```python
from build123d import *

# Parameters (mm, degrees)
SKETCH2_W                = 45
SKETCH2_H                = 62
BOSS_EXTRUDE1_DEPTH      = 5
BOSS_EXTRUDE2_DEPTH      = 10
BOSS_EXTRUDE2_DEPTH_BACK = 5
SKETCH3_W                = 55
SKETCH3_H                = 72
SKETCH3_W_2              = 45
SKETCH3_H_2              = 62
FILLET1_R                = 10


with BuildPart() as part:
    # Sketch2 → Boss-Extrude1 (new body)
    with BuildSketch(Plane(origin=(0, 0, 0), x_dir=(1, 0, 0), z_dir=(0, 1, 0))):
        with Locations((22.5, 31)):
            Rectangle(SKETCH2_W, SKETCH2_H)
    extrude(amount=BOSS_EXTRUDE1_DEPTH)

    # Sketch3 → Boss-Extrude2 (add, two sides: drawn at the far end of the back side and taken through both)
    with BuildSketch(Plane(origin=(0, 5, 0), x_dir=(1, 0, 0), z_dir=(0, 1, 0)).offset(-BOSS_EXTRUDE2_DEPTH_BACK)):
        with Locations((22.5, 31)):
            Rectangle(SKETCH3_W, SKETCH3_H)
        with Locations((22.5, 31)):
            Rectangle(SKETCH3_W_2, SKETCH3_H_2, mode=Mode.SUBTRACT)
    extrude(amount=BOSS_EXTRUDE2_DEPTH + BOSS_EXTRUDE2_DEPTH_BACK)

    # Fillet1
    fillet1_edges = [part.edges().sort_by_distance(p)[0] for p in [
        (50, 7.5, 5),
        (-5, 7.5, 5),
        (-5, 7.5, -67),
        (50, 7.5, -67),
    ]]
    fillet(fillet1_edges, radius=FILLET1_R)


solid = part.part
```
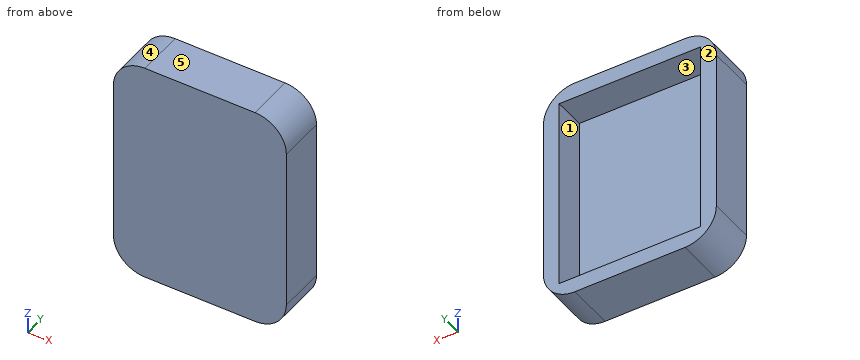
For this review, take the finished solid that the model builds, in its own axes (mm). Face numbers are marked on the shaded views. A direction names the side the tool comes from. Round coordinates to 2 decimals unless told otherwise and drop trailing zeros. Loops run counter-clockwise (first coordinate to the right, second up) from the corner with the lowest first, then second, coordinate; pieces in that order, holes last.
(1) We need section D-D (z = -63). Give the boundary of the cut face in (x, y).
Returned:
outline: (-3, 0) - (48, 0) - (48, 15) - (-3, 15) - close
(2) We need section A-A (y = 10.75). Give the boundary of the cut face in (x, z).
Returned:
outline: (-5, -57) arc R10 ccw to (5, -67) - (40, -67) arc R10 ccw to (50, -57) - (50, -5) arc R10 ccw to (40, 5) - (5, 5) arc R10 ccw to (-5, -5) - close; hole (0, -62) - (45, -62) - (45, 0) - (0, 0) - close
(3) We need section B-B (x = 35.5). Give the boundary of the cut face in (y, z).
Returned:
outline: (0, -67) - (15, -67) - (15, -62) - (5, -62) - (5, 0) - (15, 0) - (15, 5) - (0, 5) - close
(4) Tool access review of the marked faces 1 and 2: name each direction out of +Z, -Z, +X, -X, +Y, -Y from which nothing blocks a thin tool from reaching the whole face with its end or side.
Returned:
face 1: +Y
face 2: +Z, -Z, +X, -X, +Y
(5) Mouldability with a two-part tool opening along X and no side actions: class the marked faces 3, 4 and 5 as released by +X, released by -X, zero draft, split by the parting line, or undercut.
Returned:
face 3: undercut
face 4: released by -X
face 5: zero draft
(6) Clearance check with flat-ended pins moving along their axes: P1, Ø10, axis at x = 3, z = -44.5, coming from the -Y side; P2, Ø8, axis at x = 26.5, z = -13, coming from the +Y side. State where each tip first meets the part, or that it passes through.
Returned:
P1: stops at y = 0
P2: stops at y = 5
(7) Wall thickness on line 1 along X through (y, z) = (9, -21.5); line 2 along Z through (x, y) = (31, 7.5); line 3 along Y through (x, z) = (26, -52.5): over which ranges is each line inside the solid? List them lowest first.
Returned:
line 1: x = -5 to 0, 45 to 50
line 2: z = -67 to -62, 0 to 5
line 3: y = 0 to 5
(8) We need section C-C (y = 1). Give the boundary of the cut face in (x, z).
Returned:
outline: (-5, -57) arc R10 ccw to (5, -67) - (40, -67) arc R10 ccw to (50, -57) - (50, -5) arc R10 ccw to (40, 5) - (5, 5) arc R10 ccw to (-5, -5) - close
